from build123d import *

# Parameters (mm, degrees)
F0_W     = 100
F0_H     = 50
F0_W_2   = 70.7229366664
F0_H_2   = 44
F0_W_3   = 20.2770633336
F1_DEPTH = 3
F2_DEPTH = 3
F3_R     = 2.5
F4_DEPTH = 3
F5_R     = 1.25
F6_DEPTH = 25


with BuildPart() as f1:
    # F0 (on Top) → F1 (new body)
    with BuildSketch(Plane.XY):
        with Locations((-50, 25)):
            Rectangle(F0_W, F0_H)
        with Locations((-61.6385316668, 25)):
            Rectangle(F0_W_2, F0_H_2, mode=Mode.SUBTRACT)
        with Locations((-13.1385316668, 25)):
            Rectangle(F0_W_3, F0_H_2, mode=Mode.SUBTRACT)
        with Locations((-61.6385316668, 25)):
            Rectangle(F0_W_2, F0_H_2)
        with Locations((-13.1385316668, 25)):
            Rectangle(F0_W_3, F0_H_2)
    extrude(amount=F1_DEPTH)

    # F0 (on Top) → F2 (join)
    with BuildSketch(Plane.XY):
        with Locations((-61.6385316668, 25)):
            Rectangle(F0_W_2, F0_H_2)
        with Locations((-13.1385316668, 25)):
            Rectangle(F0_W_3, F0_H_2)
    extrude(amount=-F2_DEPTH)

    # F3 (on face) → F4 (cut)
    with BuildSketch(Plane.XY.offset(3)):
        with Locations((-13.1529411301, 26.6577675939)):
            Circle(F3_R)
    extrude(amount=-F4_DEPTH, mode=Mode.SUBTRACT)

    # F5 (on face) → F6 (cut)
    with BuildSketch(Plane.XY):
        with Locations((-13.1529411301, 26.6577675939)):
            Circle(F5_R)
    extrude(amount=-F6_DEPTH, mode=Mode.SUBTRACT)


solid = f1.part
The listing builds one solid part. Answer for the finished solid, in the listing's coordinates (mm). A direction names the side the tool comes from. Round coordinates to 2 decimals unless told otherwise and drop trailing zeros. Order: outer loops, then holes, each group sorted by start corner. A loop starts at its lowest first (then second) coordinate and runs counter-clockwise, first axis right, second up. Notation, with made-up numbers: (-6, 16.25) -> (48, 16.25) arc R19 ccw to (48, 21.25) -> close; hole circle Ø11 at (-35, 27). An arc over 180 degrees is marked (long way). Put each result on its own line as item: value.
Q1. Consider line 1 along X through (y, z) = (5.5, -0.7); line 2 along Y through (x, z) = (-61, -2). Determine where each line is inside the solid, lowest interval first.
Results list:
line 1: -97 to -26.28, -23.28 to -3
line 2: 3 to 47
Q2. Determine the mould class of faces 1 (the flat face through (-14, 28, 0)), 2 (the flat face through (-62, 25, -3)), 3 (the cylindrical face through (-13.424, 25.437, -1.479)), 4 (the flat face through (-62, 47, -1)) for opening direction Y: pulls with the +Y half, pulls with the -Y half, needs draft (parallel to the pull), parting line crosses it, or undercut.
Results list:
face 1: undercut
face 2: needs draft
face 3: undercut
face 4: pulls with the +Y half
Q3. Section C-C, the plane x = -93 is taken. Write down the section's boundary in (y, z).
Results list:
outline: (0, 0) -> (3, 0) -> (3, -3) -> (47, -3) -> (47, 0) -> (50, 0) -> (50, 3) -> (0, 3) -> close
Q4. Each of these flat-tipped pins is pushed along its axis until it touches: P1, Ø3.5, axis at x = -76, z = -2, coming from the -Y side; P2, Ø1.5, axis at y = 28, z = -1, coming from the -X side; P3, Ø0.9, axis at y = 26, z = -1.5, coming from the +X side. Where does it stop, or does it pass through?
Results list:
P1: y = 3
P2: x = -97
P3: x = -3
Q5. Section A-A, the plane z = -1.4 is taken. Write down the section's boundary in (x, y).
Results list:
outline: (-97, 3) -> (-26.28, 3) -> (-26.28, 47) -> (-97, 47) -> close; (-23.28, 3) -> (-3, 3) -> (-3, 47) -> (-23.28, 47) -> close; hole circle Ø2.5 at (-13.15, 26.66)
Q6. Section B-B, the plane y = 31.5 is taken. Write down the section's boundary in (x, z), and give its area (3 significant figures).
Results list:
outline: (-100, 0) -> (-97, 0) -> (-97, -3) -> (-26.28, -3) -> (-26.28, 0) -> (-23.28, 0) -> (-23.28, -3) -> (-3, -3) -> (-3, 0) -> (0, 0) -> (0, 3) -> (-100, 3) -> close
area: 573 mm^2
Q7. Which of the six approach directions +Z, -Z, +X, -X, +Y, -Y give full straight-line access (tool end or side, diameter ignored) to faces 5 (the flat face through (-26.277, 25, -1)), 6 (the flat face through (-3, 25, -1)), 7 (the flat face through (-62, 3, -1))?
Results list:
face 5: -Z, +Y, -Y
face 6: -Z, +X, +Y, -Y
face 7: -Z, +X, -X, -Y
